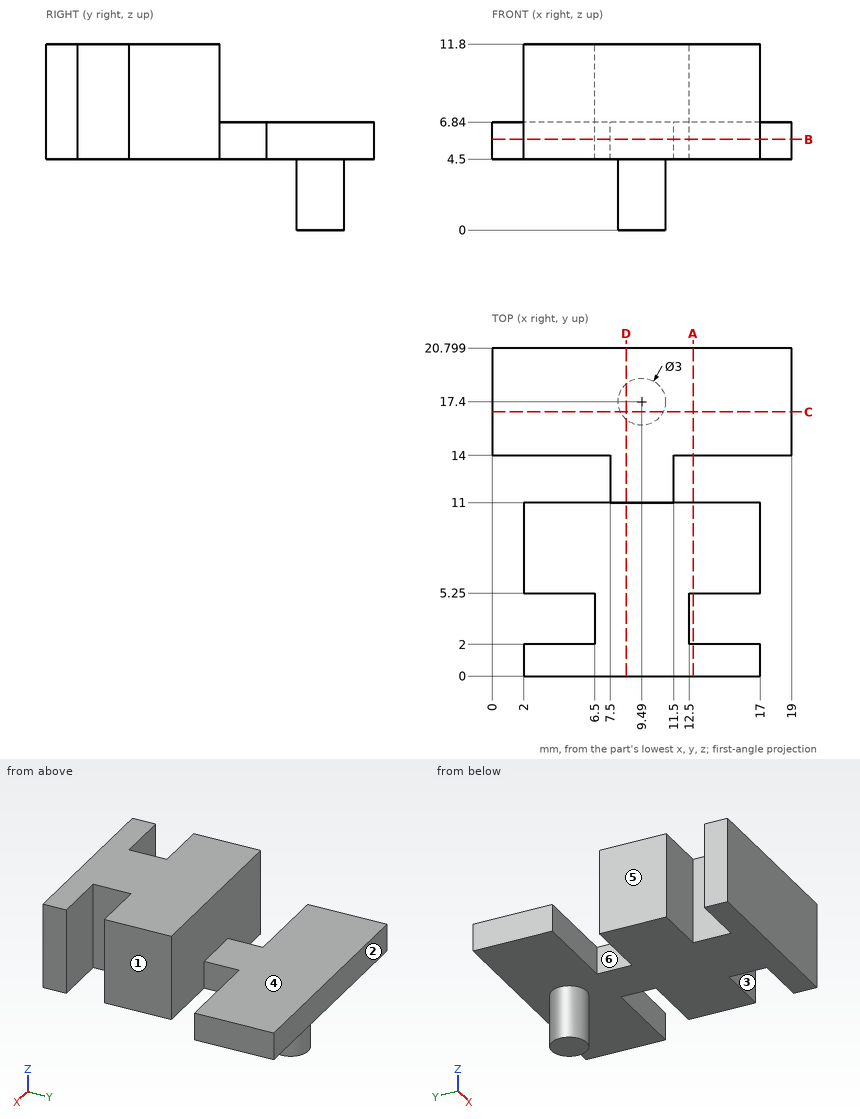
Can you work these out from the drawing? Everything is in mm from the part's minimum corner. A direction names the side the tool comes from. Round coordinates to 2 decimals unless told otherwise and drop trailing zeros. Loops run counter-clockwise (first coordinate to the right, second up) from the corner with the lowest first, then second, coordinate; pieces in that order, holes last.
1. If we section it at D-D on x = 8.5: Write out the boundary of the cut face in (y, z).
Answer list:
outline: (0, 4.5) - (16.27, 4.5) - (16.27, 0) - (18.53, 0) - (18.53, 4.5) - (20.8, 4.5) - (20.8, 6.84) - (11, 6.84) - (11, 11.8) - (0, 11.8) - close
2. If we section it at B-B on z = 5.75: Write out the boundary of the cut face in (x, y), plus the area to 3 significant figures.
Answer list:
outline: (0, 14) - (7.5, 14) - (7.5, 11) - (2, 11) - (2, 5.25) - (6.5, 5.25) - (6.5, 2) - (2, 2) - (2, 0) - (17, 0) - (17, 2) - (12.5, 2) - (12.5, 5.25) - (17, 5.25) - (17, 11) - (11.5, 11) - (11.5, 14) - (19, 14) - (19, 20.8) - (0, 20.8) - close
area: 277 mm2
3. We'd pull the mould along Y, two halves only. Please class the marked faces 1, 2 and 3: +Y half, -Y half, draft (parallel to the pull), parting line (faces both ways), or undercut.
Answer list:
face 1: draft
face 2: +Y half
face 3: undercut
4. Which directions (+Z, -Z, +X, -X, +Y, -Y) give clear straight access to the entire face, cutting with the end or side of a thin tool? Please do the marked faces 4, 5 and 6.
Answer list:
face 4: +Z, +X, -X, +Y
face 5: +Z, -Z, -X, -Y
face 6: +Z, -Z, -X
5. If I drill on line 1 along Y through (x, z) = (4.75, 6.75); line 2 along Y through (x, z) = (15.5, 9); line 3 along X through (y, z) = (7.75, 9), over which ranges is the centre line in solid material (lowest first)?
Answer list:
line 1: y = 0 to 2, 5.25 to 11, 14 to 20.8
line 2: y = 0 to 2, 5.25 to 11
line 3: x = 2 to 17
6. If we section it at A-A on x = 12.75: Write out the boundary of the cut face in (y, z).
Answer list:
outline: (0, 4.5) - (2, 4.5) - (2, 11.8) - (0, 11.8) - close; (5.25, 4.5) - (11, 4.5) - (11, 11.8) - (5.25, 11.8) - close; (14, 4.5) - (20.8, 4.5) - (20.8, 6.84) - (14, 6.84) - close
7. If we section it at C-C on y = 16.75: Write out the boundary of the cut face in (x, z).
Answer list:
outline: (0, 4.5) - (8.14, 4.5) - (8.14, 0) - (10.84, 0) - (10.84, 4.5) - (19, 4.5) - (19, 6.84) - (0, 6.84) - close
8. For P1, Ø6, axis at x = 14, y = 13.5, coming from the -Z side; P2, Ø1.6, axis at y = 4.5, z = 9, coming from the +X side; P3, Ø1.6, axis at y = 0.5, z = 7, coming from the -X side, each with a flat end and sliding along its axis, tell me the tip position at first contact or that it passes through.
Answer list:
P1: stops at z = 4.5
P2: stops at x = 17
P3: stops at x = 2
